```python
from build123d import *

# Parameters (mm, degrees)
SKETCH2_W                = 6.223
SKETCH2_H                = 12.7
BOSS_EXTRUDE1_DEPTH      = 19.3294
SKETCH3_R                = 1.905
CUT_EXTRUDE1_DEPTH       = 19.3294
BOSS_EXTRUDE2_DEPTH      = 8.89
BOSS_EXTRUDE2_DEPTH_BACK = 22.86
CUT_EXTRUDE2_START       = -7.62
CUT_EXTRUDE2_DEPTH       = 6.35
FILLET1_R                = 1.27


with BuildPart() as part:
    # Sketch2 → Boss-Extrude1 (new body)
    with BuildSketch(Plane.XY):
        with Locations((3.1115, 6.35)):
            Rectangle(SKETCH2_W, SKETCH2_H)
    extrude(amount=BOSS_EXTRUDE1_DEPTH)

    # Sketch3 → Cut-Extrude1 (cut)
    with BuildSketch(Plane(origin=(6.223, 0, 0), x_dir=(0, 0, -1), z_dir=(1, 0, 0))):
        with Locations(Location((-14.8844, 8.382, 0), (0, 0, 90))):
            Circle(SKETCH3_R)
        with Locations(Location((-5.1054, 8.382, 0), (0, 0, 90))):
            Circle(SKETCH3_R)
    extrude(amount=-CUT_EXTRUDE1_DEPTH, mode=Mode.SUBTRACT)

    # Sketch4 → Boss-Extrude2 (add, two sides: drawn at the far end of the back side and taken through both)
    with BuildSketch(Plane(origin=(0, 12.7, 0), x_dir=(1, 0, 0), z_dir=(0, 1, 0)).offset(-BOSS_EXTRUDE2_DEPTH_BACK)):
        with BuildLine():
            Line((6.223, 3.81), (6.223, 0))
            Line((6.223, 0), (0, 0))
            Line((0, 0), (0, 3.81))
            ThreePointArc((0, 3.81), (3.1115, 2.995437449), (6.223, 3.81))
        make_face()
    extrude(amount=BOSS_EXTRUDE2_DEPTH + BOSS_EXTRUDE2_DEPTH_BACK)

    # Sketch5 → Cut-Extrude2 (cut)
    with BuildSketch(Plane(origin=(0, 21.59, 0), x_dir=(1, 0, 0), z_dir=(0, 1, 0)).offset(CUT_EXTRUDE2_START)):
        with BuildLine():
            Line((5.715, 0.508), (5.715, 3.000837245))
            Line((5.715, 3.000837245), (5.715, 3.553694382))
            ThreePointArc((5.715, 3.553694382), (5.971872247, 3.676154372), (6.223, 3.81))
            Line((6.223, 3.81), (6.223, 0))
            Line((6.223, 0), (0, 0))
            Line((0, 0), (0, 3.81))
            ThreePointArc((0, 3.81), (0.251127753, 3.676154372), (0.508, 3.553694382))
            Line((0.508, 3.553694382), (0.508, 3.000837245))
            Line((0.508, 3.000837245), (0.508, 0.508))
            Line((0.508, 0.508), (5.715, 0.508))
        make_face()
    cut_extrude2 = extrude(amount=CUT_EXTRUDE2_DEPTH, mode=Mode.SUBTRACT)

    # Mirror1: Cut-Extrude2 across plane
    add(cut_extrude2.mirror(Plane.ZX.offset(5.715)), mode=Mode.SUBTRACT)

    # Fillet1
    fillet1_edges = [part.edges().sort_by_distance(p)[0] for p in [
        (6.223, 13.335, 0),
        (6.223, -9.525, 0),
        (0, -9.525, 0),
        (0, 13.335, 0),
        (6.223, 20.955, 0),
        (0, 20.955, 0),
        (0.508, 17.145, -0.508),
        (5.715, 17.145, -0.508),
        (0, -1.27, 0),
        (6.223, -1.27, 0),
        (5.715, -5.715, -0.508),
        (0.508, -5.715, -0.508),
    ]]
    fillet(fillet1_edges, radius=FILLET1_R)


solid = part.part
```
Can you work these out from the model? Positions are in its coordinate system, mm. A direction names the side the tool comes from. Coordinates: 2 decimals unless noted, no trailing zeros. Order: outer loops, then holes, each group sorted by start corner. A loop starts at its lowest first (then second) coordinate and runs counter-clockwise, first axis right, second up. Notation, with made-up numbers: (0, -5.75) - (5, -5.75) arc R14 cw to (5, 10.25) - close; hole circle Ø4 at (-6, 45.25). An arc over 180 degrees is marked (long way). Answer in a Markdown table with one row per item.
1. If we mould it in two halves opening along Z, with no side actions, what happens to faces 6 (the flat face through (3, 21, 0)), 7 (the cylindrical face through (3.155, 7.969, 3.246)), 8 (the flat face through (3.1, 20.32, -0.2)), 9 (the cylindrical face through (3.066, 5.493, -2.996))? For each: pulls with the +Z half, pulls with the -Z half, needs draft (parallel to the pull), parting line crosses it, or undercut.
Reply:
| item | result |
|---|---|
| face 6 | pulls with the +Z half |
| face 7 | undercut |
| face 8 | needs draft |
| face 9 | pulls with the -Z half |
2. Suppose I cut it at C-C (y = 13.5). Please give me the cut outline in (x, z), and give its area (3 significant figures).
Reply:
| item | result |
|---|---|
| outline | (0, -3.81) arc R6.35 cw to (6.22, -3.81) - (6.22, -1.27) arc R1.27 ccw to (4.95, 0) - (1.27, 0) arc R1.27 ccw to (0, -1.27) - close |
| area | 19.6 mm^2 |
3. Suppose I cut it at D-D (z = 7.5). Please give me the cut outline in (x, y), and give its area (3 significant figures).
Reply:
| item | result |
|---|---|
| outline | (0, 0) - (6.22, 0) - (6.22, 12.7) - (0, 12.7) - close |
| area | 79.0 mm^2 |
4. For pin 1 (1.4 mm diameter, centred on x = 3, y = 21, fed in from +Z); pin 2 (2 mm diameter, centred on x = 3, y = 16, fed in from +Z); pin 3 (1.5 mm diameter, centred on x = 4.5, y = 6, fed in from -Z); pin 4 (1 mm diameter, centred on x = 2.5, y = 13, fed in from +Z), each with a flat end and sliding along its axis, tell me the tip position at first contact or that it passes through.
Reply:
| item | result |
|---|---|
| pin 1 | stops at z = 0 |
| pin 2 | stops at z = -0.51 |
| pin 3 | stops at z = -3.37 |
| pin 4 | stops at z = 19.33 |
5. Suppose I cut it at B-B (x = 2.75). Please give me the cut outline in (y, z) (3 decimals).
Reply:
| item | result |
|---|---|
| outline | (-10.16, -3.006) - (21.59, -3.006) - (21.59, 0) - (20.32, 0) - (20.32, -0.508) - (13.97, -0.508) - (13.97, 0) - (12.7, 0) - (12.7, 19.329) - (0, 19.329) - (0, 0) - (-2.54, 0) - (-2.54, -0.508) - (-8.89, -0.508) - (-8.89, 0) - (-10.16, 0) - close; hole circle Ø3.81 at (8.382, 5.105); hole circle Ø3.81 at (8.382, 14.884) |
6. For faces 1 (the flat face through (3, 13, 0)), 2 (the flat face through (0.508, -6, -3)), 3 (the flat face through (5.715, 17, -3)), 4 (the cylindrical face through (5.86, -9.52, -0.38)), 5 (the cylindrical face through (0.362, 13.344, -0.382)), which set-ups out of +Z, -Z, +X, -X, +Y, -Y let a thin tool reach every point of the face, with its end or its side?
Reply:
| item | result |
|---|---|
| face 1 | +Z, +X, -X, +Y |
| face 2 | +Z, -Z, -X |
| face 3 | +Z, -Z, +X |
| face 4 | +Z, +X, -Y |
| face 5 | +Z, -X, +Y |
7. If I drill on line 1 along Y through (x, z) = (1, 15); line 2 along Y through (x, z) = (1.5, 2.5); line 3 along Z through (x, y) = (6, 9), over which ranges is the centre line in solid material (lowest first)?
Reply:
| item | result |
|---|---|
| line 1 | y = 0 to 6.48, 10.28 to 12.7 |
| line 2 | y = 0 to 12.7 |
| line 3 | z = -3.69 to 3.3, 6.91 to 13.08, 16.69 to 19.33 |
8. Suppose I cut it at A-A (z = 13.75). Please give me the cut outline in (x, y).
Reply:
| item | result |
|---|---|
| outline | (0, 0) - (6.22, 0) - (6.22, 6.85) - (0, 6.85) - close; (0, 9.91) - (6.22, 9.91) - (6.22, 12.7) - (0, 12.7) - close |
